```python
from build123d import *

# Parameters (mm, degrees)
F0_R     = 63.625
F1_DEPTH = 2
F2_R     = 0.75
F3_DEPTH = 1


with BuildPart() as f1:
    # F0 (on Top) → F1 (new body)
    with BuildSketch(Plane.XY):
        Circle(F0_R)
    extrude(amount=F1_DEPTH)

    # F2 (on face) → F3 (join)
    with BuildSketch(Plane.XY.offset(2)):
        with Locations((0, 60)):
            Circle(F2_R)
        with Locations((-60, 0)):
            Circle(F2_R)
        with Locations((0, -60)):
            Circle(F2_R)
        with Locations((60, 0)):
            Circle(F2_R)
    extrude(amount=F3_DEPTH)


solid = f1.part
```
Geometry: final body of the model. Coordinates: model frame, mm. Coordinates: 2 decimals unless noted, no trailing zeros. Order: outer loops, then holes, each group sorted by start corner. A loop starts at its lowest first (then second) coordinate and runs counter-clockwise, first axis right, second up. Notation, with made-up numbers: M -30.5,24.25 L -1.5,24.25 A32 ccw -1.5,63.25 Z; hole C 49,28.25 d1. An arc over 180 degrees is marked long. Answer in a Markdown table with one row per item. Add a question column.
Q1. Section query C-C on y = 12. Return the cut outline in (x, z), and give its area (3 significant figures).
Q2. Line query: L1, parallel to Z at x = -47.5, y = 6; L2, parallel to X at y = 27, z = 1.75; L3, parallel to X at y = -10.5, z = 0.4. Output: solid intervals per line, ascending.
Q3. Section query A-A on z = 1.2. Return the cut outline in (x, y) (3 decimals), and give its area (3 significant figures).
Q4. Section query B-B on x = 2.5. Return the cut outline in (y, z).
Q5. Contact query for a flat-ended pin moving along its axis: P1, Ø12, axis at x = -39, y = 1.5, coming from the +Z side. Output: stop coordinate, or through.
Completed:
| question | item | result |
|---|---|---|
| 1 | outline | M -62.48,0 L 62.48,0 L 62.48,2 L -62.48,2 Z |
| 1 | area | 250 mm2 |
| 2 | L1 | z = 0 to 2 |
| 2 | L2 | x = -57.61 to 57.61 |
| 2 | L3 | x = -62.75 to 62.75 |
| 3 | outline | C 0,0 d127.25 |
| 3 | area | 12,700 mm2 |
| 4 | outline | M -63.58,0 L 63.58,0 L 63.58,2 L -63.58,2 Z |
| 5 | P1 | stops at z = 2 |
